The model under review builds one solid part; all positions refer to its coordinate system, in mm. Round coordinates to 2 decimals unless told otherwise and drop trailing zeros. Return JSON: item names as keys, results as strings. Group by question number.
from build123d import *

# Parameters (mm, degrees)
F0_W      = 25.4
F0_H      = 25.4
F0_W_2    = 1803.4
F0_H_2    = 584.2
F1_DEPTH  = 25.4
F2_W      = 1841.5
F2_H      = 622.3
F2_W_2    = 1803.4
F2_H_2    = 584.2
F3_DEPTH  = 19.05
F4_W      = 25.4
F4_H      = 232.57764
F4_H_2    = 25.4
F4_W_2    = 69.8373
F4_H_3    = 68.24472
F5_DEPTH  = 25.4
F6_W      = 19.05
F6_H      = 251.62764
F6_W_2    = 107.9373
F6_H_2    = 106.34472
F6_W_3    = 69.8373
F6_H_3    = 68.24472
F7_DEPTH  = 19.05
F8_R      = 3.571875
F9_DEPTH  = 25.4
F10_R     = 3.5687
F11_DEPTH = 25.4
F12_W     = 6.35
F12_H     = 622.3
F13_DEPTH = 25.4


# Not quite as in the source:
# - a feature names something its author has since deleted; it is built from what else it names


with BuildPart() as f1:
    # F0 (on Top) → F1 (new body)
    with BuildSketch(Plane.XY):
        with Locations((12.7, -12.7)):
            Rectangle(F0_W, F0_H)
        with Locations((927.1, -12.7)):
            Rectangle(F0_W_2, F0_H)
        with Locations((12.7, -317.5)):
            Rectangle(F0_W, F0_H_2)
        with Locations((1841.5, -12.7)):
            Rectangle(F0_W, F0_H)
        with Locations((12.7, -622.3)):
            Rectangle(F0_W, F0_H)
        with Locations((1841.5, -317.5)):
            Rectangle(F0_W, F0_H_2)
        with Locations((927.1, -622.3)):
            Rectangle(F0_W_2, F0_H)
        with Locations((1841.5, -622.3)):
            Rectangle(F0_W, F0_H)
    extrude(amount=F1_DEPTH)

    # F2 (on face) → F3 (cut)
    with BuildSketch(Plane.XY.offset(25.4)):
        with Locations((927.1, -317.5)):
            Rectangle(F2_W, F2_H)
        with Locations((927.1, -317.5)):
            Rectangle(F2_W_2, F2_H_2, mode=Mode.SUBTRACT)
    extrude(amount=-F3_DEPTH, mode=Mode.SUBTRACT)

    # F4 (on face) → F5 (join)
    with BuildSketch(Plane(origin=(0, 0, 0), x_dir=(1, 0, 0), z_dir=(0, 0, -1))):
        with Locations((466.2932, 493.31118)):
            Rectangle(F4_W, F4_H)
        with Locations((466.2932, 622.3)):
            Rectangle(F4_W, F4_H_2)
        with Locations((561.5305, 622.3)):
            Rectangle(F4_W, F4_H_2)
        with Locations((561.5305, 493.31118)):
            Rectangle(F4_W, F4_H)
        with Locations((561.5305, 364.32236)):
            Rectangle(F4_W, F4_H_2)
        with Locations((513.91185, 364.32236)):
            Rectangle(F4_W_2, F4_H_2)
        with Locations((466.2932, 364.32236)):
            Rectangle(F4_W, F4_H_2)
        with Locations((466.2932, 317.5)):
            Rectangle(F4_W, F4_H_3)
        with Locations((561.5305, 317.5)):
            Rectangle(F4_W, F4_H_3)
        with Locations((561.5305, 270.67764)):
            Rectangle(F4_W, F4_H_2)
        with Locations((513.91185, 270.67764)):
            Rectangle(F4_W_2, F4_H_2)
        with Locations((466.2932, 270.67764)):
            Rectangle(F4_W, F4_H_2)
        with Locations((466.2932, 141.68882)):
            Rectangle(F4_W, F4_H)
        with Locations((466.2932, 12.7)):
            Rectangle(F4_W, F4_H_2)
        with Locations((561.5305, 12.7)):
            Rectangle(F4_W, F4_H_2)
        with Locations((561.5305, 141.68882)):
            Rectangle(F4_W, F4_H)
        with Locations((1292.6568, 317.5)):
            Rectangle(F4_W, F4_H_3)
        with Locations((1292.6568, 622.3)):
            Rectangle(F4_W, F4_H_2)
        with Locations((1387.8941, 622.3)):
            Rectangle(F4_W, F4_H_2)
        with Locations((1292.6568, 493.31118)):
            Rectangle(F4_W, F4_H)
        with Locations((1387.8941, 493.31118)):
            Rectangle(F4_W, F4_H)
        with Locations((1340.27545, 364.32236)):
            Rectangle(F4_W_2, F4_H_2)
        with Locations((1387.8941, 317.5)):
            Rectangle(F4_W, F4_H_3)
        with Locations((1387.8941, 364.32236)):
            Rectangle(F4_W, F4_H_2)
        with Locations((1292.6568, 364.32236)):
            Rectangle(F4_W, F4_H_2)
        with Locations((1292.6568, 270.67764)):
            Rectangle(F4_W, F4_H_2)
        with Locations((1340.27545, 270.67764)):
            Rectangle(F4_W_2, F4_H_2)
        with Locations((1387.8941, 270.67764)):
            Rectangle(F4_W, F4_H_2)
        with Locations((1387.8941, 141.68882)):
            Rectangle(F4_W, F4_H)
        with Locations((1292.6568, 141.68882)):
            Rectangle(F4_W, F4_H)
        with Locations((1292.6568, 12.7)):
            Rectangle(F4_W, F4_H_2)
        with Locations((1387.8941, 12.7)):
            Rectangle(F4_W, F4_H_2)
    extrude(amount=-F5_DEPTH)

    # F6 (on face) → F7 (cut)
    with BuildSketch(Plane.XY.offset(25.4)):
        with Locations((1295.8318, -132.16382)):
            Rectangle(F6_W, F6_H)
        with Locations((1384.7191, -132.16382)):
            Rectangle(F6_W, F6_H)
        with Locations((1340.27545, -317.5)):
            Rectangle(F6_W_2, F6_H_2)
        with Locations((1340.27545, -317.5)):
            Rectangle(F6_W_3, F6_H_3, mode=Mode.SUBTRACT)
        with Locations((1384.7191, -502.83618)):
            Rectangle(F6_W, F6_H)
        with Locations((1295.8318, -502.83618)):
            Rectangle(F6_W, F6_H)
        with Locations((558.3555, -502.83618)):
            Rectangle(F6_W, F6_H)
        with Locations((469.4682, -502.83618)):
            Rectangle(F6_W, F6_H)
        with Locations((513.91185, -317.5)):
            Rectangle(F6_W_2, F6_H_2)
        with Locations((513.91185, -317.5)):
            Rectangle(F6_W_3, F6_H_3, mode=Mode.SUBTRACT)
        with Locations((469.4682, -132.16382)):
            Rectangle(F6_W, F6_H)
        with Locations((558.3555, -132.16382)):
            Rectangle(F6_W, F6_H)
    extrude(amount=-F7_DEPTH, mode=Mode.SUBTRACT)

    # F8 (on face) → F9 (cut)
    with BuildSketch(Plane(origin=(0, 0, 0), x_dir=(1, 0, 0), z_dir=(0, 0, -1))):
        with Locations((12.7, 622.3)):
            Circle(F8_R)
        with Locations((622.3, 622.3)):
            Circle(F8_R)
        with Locations((1231.9, 622.3)):
            Circle(F8_R)
        with Locations((1841.5, 622.3)):
            Circle(F8_R)
    extrude(amount=-F9_DEPTH, mode=Mode.SUBTRACT)

    # F10 (on face) → F11 (cut)
    with BuildSketch(Plane(origin=(0, 0, 0), x_dir=(-1, 0, 0), z_dir=(0, 1, 0))):
        with Locations((-1841.5, 12.7)):
            Circle(F10_R)
        with Locations((-1231.9, 12.7)):
            Circle(F10_R)
        with Locations((-622.3, 12.7)):
            Circle(F10_R)
        with Locations((-12.7, 12.7)):
            Circle(F10_R)
    extrude(amount=-F11_DEPTH, mode=Mode.SUBTRACT)

    # F12 (on face) → F13 (join)
    with BuildSketch(Plane.XY.offset(25.4)):
        Polygon((230.3526, -6.35), (229.5906, -6.35), (224.0026, -6.35), (224.0026, -628.65), (229.5906, -628.65), (230.3526, -628.65), align=None)
        with Locations((930.26865, -317.5)):
            Rectangle(F12_W, F12_H)
        with Locations((1621.4471, -317.5)):
            Rectangle(F12_W, F12_H)
    extrude(amount=-F13_DEPTH)


solid = f1.part
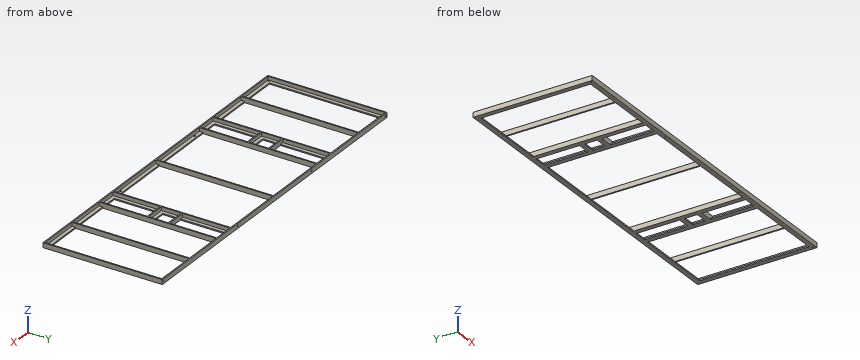
Item 1: Consider section A-A on y = -95. Give the number of separate pieces and of enclosed holes in the cut face, plus the area to 3 significant figures.
Item 2: Wall thickness on line 1 along X through (y, z) = (-622.3, 2); line 2 along Y through (x, z) = (462.5, 23.25); line 3 along Y through (x, z) = (1231.9, 4.5): over which ranges is each line inside the solid? List them lowest first.
Item 3: Insertion check: pin 1 Ø3 at (x, y) = (1377, -100) entering from +Z; pin 2 Ø9.5 at (x, z) = (622.3, 12.7) entering from +Y. Each pin has a flat end and moves straight along its axis. Give the tip position at first contact, or say it passes through.
Values:
{
 "1": {"separate pieces": "9", "enclosed holes": "0", "area": "2,180 mm^2"},
 "2": {"line 1": "0 to 9.13, 16.27 to 618.73, 625.87 to 1228.33, 1235.47 to 1837.93, 1845.07 to 1854.2", "line 2": "-635 to -628.65, -377.02 to -370.67, -264.33 to -257.98, -6.35 to 0", "line 3": "-635 to -625.87, -618.73 to -609.6, -25.4 to 0"},
 "3": {"pin 1": "z = 6.35", "pin 2": "y = 0"}
}
